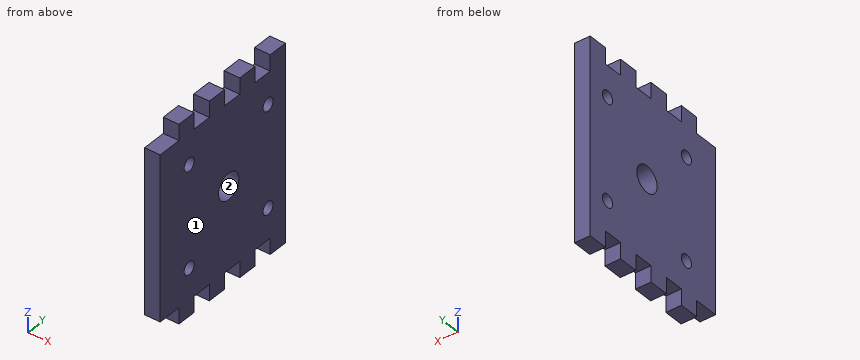
```python
from build123d import *

# Parameters (mm, degrees)
SKETCH1_W               = 76.2
SKETCH1_H               = 62.738
BOSS_EXTRUDE1_DEPTH     = 6.096
SKETCH2_R               = 5.08
SKETCH2_R_2             = 2.54
CUT_EXTRUDE1_DEPTH      = 6.096
SKETCH3_W               = 6.223
SKETCH3_H               = 7.62
CUT_EXTRUDE2_DEPTH      = 6.096
CUT_EXTRUDE3_DEPTH      = 7.874
CUT_EXTRUDE3_DEPTH_BACK = 6.096
SKETCH4_W               = 6.223
SKETCH4_H               = 9.398


with BuildPart() as part:
    # Sketch1 → Boss-Extrude1 (new body)
    with BuildSketch(Plane(origin=(0, 0, 0), x_dir=(0, 0, -1), z_dir=(1, 0, 0))):
        with Locations((1.357482185, -4.852847981)):
            Rectangle(SKETCH1_W, SKETCH1_H)
    extrude(amount=BOSS_EXTRUDE1_DEPTH)

    # Sketch2 → Cut-Extrude1 (cut)
    with BuildSketch(Plane(origin=(6.096, 0, 0), x_dir=(0, 0, -1), z_dir=(1, 0, 0))):
        with Locations((1.357482185, -1.931847981)):
            Circle(SKETCH2_R)
        with Locations((-18.399081281, 17.824715485)):
            Circle(SKETCH2_R_2)
        with Locations((21.114045652, 17.824715485)):
            Circle(SKETCH2_R_2)
        with Locations((21.114045652, -21.688411447)):
            Circle(SKETCH2_R_2)
        with Locations((-18.399081281, -21.688411447)):
            Circle(SKETCH2_R_2)
    extrude(amount=-CUT_EXTRUDE1_DEPTH, mode=Mode.SUBTRACT)

    # Sketch3 → Cut-Extrude2 (cut)
    with BuildSketch(Plane(origin=(6.096, 0, 0), x_dir=(0, 0, -1), z_dir=(1, 0, 0))):
        with Locations((-33.631017815, 15.086152019)):
            Rectangle(SKETCH3_W, SKETCH3_H)
        with Locations((-33.631017815, -0.153847981)):
            Rectangle(SKETCH3_W, SKETCH3_H)
        with Locations((-33.631017815, -15.393847981)):
            Rectangle(SKETCH3_W, SKETCH3_H)
        with Locations((36.345982185, -15.393847981)):
            Rectangle(SKETCH3_W, SKETCH3_H)
        with Locations((36.345982185, 15.086152019)):
            Rectangle(SKETCH3_W, SKETCH3_H)
        with Locations((36.345982185, -0.153847981)):
            Rectangle(SKETCH3_W, SKETCH3_H)
    extrude(amount=-CUT_EXTRUDE2_DEPTH, mode=Mode.SUBTRACT)

    # Sketch4 → Cut-Extrude3 (cut, two sides: drawn at the far end of the back side and taken through both)
    with BuildSketch(Plane(origin=(6.096, 0, 0), x_dir=(0, 0, -1), z_dir=(1, 0, 0)).offset(-CUT_EXTRUDE3_DEPTH_BACK)):
        with Locations((36.345982185, -31.522847981)):
            Rectangle(SKETCH4_W, SKETCH4_H)
        with Locations((-33.631017815, -31.522847981)):
            Rectangle(SKETCH4_W, SKETCH4_H)
    extrude(amount=CUT_EXTRUDE3_DEPTH + CUT_EXTRUDE3_DEPTH_BACK, mode=Mode.SUBTRACT)


solid = part.part
```
Design review of the part built by this model. Coordinates are the model's own, in mm. Face numbers are marked on the shaded views. Give positions to 0.01 mm unless a question says otherwise; leave off trailing zeros. Order: outer loops, then holes, each group sorted by start corner. A loop starts at its lowest first (then second) coordinate and runs counter-clockwise, first axis right, second up. Notation, with made-up numbers: (13, -26.5) - (27, -26.5) arc R26 cw to (27, 10.5) - close; hole circle Ø11 at (81.25, -4). An arc over 180 degrees is marked (long way). Use a Markdown table: item, result. Add a question column.
(1) Clearance check with flat-ended pins moving along their axes: P1, Ø1.8, axis at x = 3, y = 1, coming from the +Z side; P2, Ø1.8, axis at x = 3.5, y = -30.5, coming from the -Z side; P3, Ø3, axis at x = 2.5, z = 32.5, coming from the -Y side; P4, Ø6, axis at y = -1.93, z = -1.36, coming from the +X side (3 decimals). State where each tip first meets the part, or that it passes through.
(2) Add section B-B on z = 0. Give the boundary of the cut face in (x, y), then the cut area to 3 significant figures.
(3) Add section A-A on y = -20.5. Give the boundary of the cut face in (x, z), then the cut area to 3 significant figures.
(4) Add section C-C on y = 2. Give the boundary of the cut face in (x, z), then the cut area to 3 significant figures.
(5) Wall thickness on probe 1 along Z at (x, y) = (3, -21.5); probe 2 along Y at (x, z) = (1.75, 32); probe 3 along Y at (x, z) = (0.5, -1): over which ranges is each line inside the solid? List them lowest first. Write a range as [from, to].
(6) Add section D-D on y = -28. Give the boundary of the cut face in (x, z).
(7) Mouldability with a two-part tool opening along Y and no side actions: class the marked faces 1 and 2 as +Y half, -Y half, draft (parallel to the pull), parting line (faces both ways), or undercut.
Report:
| question | item | result |
|---|---|---|
| 1 | P1 | stops at z = 30.52 |
| 1 | P2 | stops at z = -33.23 |
| 1 | P3 | stops at y = -26.82 |
| 1 | P4 | passes through |
| 2 | outline | (0, -36.22) - (6.1, -36.22) - (6.1, -6.83) - (0, -6.83) - close; (0, 2.96) - (6.1, 2.96) - (6.1, 26.52) - (0, 26.52) - close |
| 2 | area | 323 mm² |
| 3 | outline | (0, -39.46) - (6.1, -39.46) - (6.1, -23.36) - (0, -23.36) - close; (0, -18.87) - (6.1, -18.87) - (6.1, 16.15) - (0, 16.15) - close; (0, 20.64) - (6.1, 20.64) - (6.1, 36.74) - (0, 36.74) - close |
| 3 | area | 410 mm² |
| 4 | outline | (0, -33.23) - (6.1, -33.23) - (6.1, -4.57) - (0, -4.57) - close; (0, 1.86) - (6.1, 1.86) - (6.1, 30.52) - (0, 30.52) - close |
| 4 | area | 349 mm² |
| 5 | probe 1 | z = [-39.46, -23.65], [-18.58, 15.87], [20.93, 36.74] |
| 5 | probe 2 | y = [-26.82, -19.2], [-11.58, -3.96], [3.66, 11.28], [18.9, 26.52] |
| 5 | probe 3 | y = [-36.22, -7], [3.14, 26.52] |
| 6 | outline | (0, -33.23) - (6.1, -33.23) - (6.1, 30.52) - (0, 30.52) - close |
| 7 | face 1 | draft |
| 7 | face 2 | undercut |
